Source: CAD feature listing. Evaluate the final solid. Frame: model axes, mm. A direction names the side the tool comes from. Give positions to 0.01 mm unless a question says otherwise; leave off trailing zeros. Write each loop counter-clockwise with the first axis right and the second up, starting at its lowest first coordinate (ties: lowest second). Pieces come first, ordered by that corner, then holes. Notation, with made-up numbers: M 72.25,65.5 L 76.25,65.5 A33 cw 76.25,98.5 Z; hole C 47.5,-20.75 d8. An arc over 180 degrees is marked long. Return JSON: item names as keys, results as strings.
```python
from build123d import *

# Parameters (mm, degrees)
SKETCH1_W           = 110
SKETCH1_H           = 30
BOSS_EXTRUDE1_DEPTH = 12
FILLET2_R           = 8
SKETCH4_R           = 6.5
CUT_EXTRUDE1_DEPTH  = 67.870108383
SKETCH3_W           = 23
SKETCH3_H           = 13
CUT_EXTRUDE2_DEPTH  = 10
SKETCH5_W           = 32
SKETCH5_H           = 18
CUT_EXTRUDE3_DEPTH  = 1.5
FILLET4_R           = 3
SKETCH8_R           = 6.5
CUT_EXTRUDE4_DEPTH  = 63.574437799
SKETCH10_W          = 23
SKETCH10_H          = 13
CUT_EXTRUDE5_DEPTH  = 10
SKETCH12_W          = 32
SKETCH12_H          = 18
CUT_EXTRUDE6_DEPTH  = 1.5
FILLET5_R           = 3
SKETCH14_R          = 1
CUT_EXTRUDE7_DEPTH  = 4
SKETCH6_R           = 1
CUT_EXTRUDE8_DEPTH  = 5


with BuildPart() as part:
    # Sketch1 → Boss-Extrude1 (new body)
    with BuildSketch(Plane(origin=(0, 0, 0), x_dir=(1, 0, 0), z_dir=(0, 1, 0))):
        with Locations((8.243243243, 3.108108108)):
            Rectangle(SKETCH1_W, SKETCH1_H)
    extrude(amount=BOSS_EXTRUDE1_DEPTH)

    # Fillet2
    fillet2_edges = [part.edges().sort_by_distance(p)[0] for p in [
        (-46.756756757, 6, -18.108108108),
        (63.243243243, 6, -18.108108108),
        (63.243243243, 6, 11.891891892),
        (-46.756756757, 6, 11.891891892),
    ]]
    fillet(fillet2_edges, radius=FILLET2_R)

    # Sketch4 → Cut-Extrude1 (cut, through all)
    with BuildSketch(Plane(origin=(0, 12, 0), x_dir=(1, 0, 0), z_dir=(0, 1, 0))):
        with Locations(Location((-27.929103529, 3.108108108, 0), (0, 0, 270))):
            Circle(SKETCH4_R)
    extrude(amount=-CUT_EXTRUDE1_DEPTH, mode=Mode.SUBTRACT)

    # Sketch3 → Cut-Extrude2 (cut)
    with BuildSketch(Plane(origin=(0, 12, 0), x_dir=(1, 0, 0), z_dir=(0, 1, 0))):
        with Locations((-23.179103529, 3.108108108)):
            Rectangle(SKETCH3_W, SKETCH3_H)
    extrude(amount=-CUT_EXTRUDE2_DEPTH, mode=Mode.SUBTRACT)

    # Sketch5 → Cut-Extrude3 (cut)
    with BuildSketch(Plane(origin=(0, 12, 0), x_dir=(1, 0, 0), z_dir=(0, 1, 0))):
        with Locations((-23.262280593, 3.273133416)):
            Rectangle(SKETCH5_W, SKETCH5_H)
    extrude(amount=-CUT_EXTRUDE3_DEPTH, mode=Mode.SUBTRACT)

    # Fillet4
    fillet4_edges = [part.edges().sort_by_distance(p)[0] for p in [
        (-39.262280593, 11.25, 5.726866584),
        (-39.262280593, 11.25, -12.273133416),
        (-7.262280593, 11.25, -12.273133416),
        (-7.262280593, 11.25, 5.726866584),
    ]]
    fillet(fillet4_edges, radius=FILLET4_R)

    # Sketch8 → Cut-Extrude4 (cut, through all)
    with BuildSketch(Plane(origin=(11.720616789, 0, 0.652410252), x_dir=(-1, 0, 0), z_dir=(0, -1, 0))):
        with Locations(Location((-27.929103529, 3.108108108, 0), (0, 0, 90))):
            Circle(SKETCH8_R)
    extrude(amount=-CUT_EXTRUDE4_DEPTH, mode=Mode.SUBTRACT)

    # Sketch10 → Cut-Extrude5 (cut)
    with BuildSketch(Plane(origin=(11.720616789, 0, 0.652410252), x_dir=(-1, 0, 0), z_dir=(0, -1, 0))):
        with Locations((-23.179103529, 3.108108108)):
            Rectangle(SKETCH10_W, SKETCH10_H)
    extrude(amount=-CUT_EXTRUDE5_DEPTH, mode=Mode.SUBTRACT)

    # Sketch12 → Cut-Extrude6 (cut)
    with BuildSketch(Plane(origin=(11.720616789, 0, 0.652410252), x_dir=(-1, 0, 0), z_dir=(0, -1, 0))):
        with Locations((-23.262280593, 3.273133416)):
            Rectangle(SKETCH12_W, SKETCH12_H)
    extrude(amount=-CUT_EXTRUDE6_DEPTH, mode=Mode.SUBTRACT)

    # Fillet5
    fillet5_edges = [part.edges().sort_by_distance(p)[0] for p in [
        (50.982897382, 0.75, 6.379276835),
        (50.982897382, 0.75, -11.620723165),
        (18.982897382, 0.75, -11.620723165),
        (18.982897382, 0.75, 6.379276835),
    ]]
    fillet(fillet5_edges, radius=FILLET5_R)

    # Sketch14 → Cut-Extrude7 (cut)
    with BuildSketch(Plane(origin=(11.720616789, 1.5, 0.652410252), x_dir=(-1, 0, 0), z_dir=(0, -1, 0))):
        with Locations(Location((-37.179103529, 3.108108108, 0), (0, 0, 90))):
            Circle(SKETCH14_R)
        with Locations(Location((-9.179103529, 3.108108108, 0), (0, 0, 270))):
            Circle(SKETCH14_R)
    extrude(amount=-CUT_EXTRUDE7_DEPTH, mode=Mode.SUBTRACT)

    # Sketch6 → Cut-Extrude8 (cut)
    with BuildSketch(Plane(origin=(0, 10.5, 0), x_dir=(1, 0, 0), z_dir=(0, 1, 0))):
        with Locations(Location((-37.179103529, 3.108108108, 0), (0, 0, 270))):
            Circle(SKETCH6_R)
        with Locations(Location((-9.179103529, 3.108108108, 0), (0, 0, 90))):
            Circle(SKETCH6_R)
    extrude(amount=-CUT_EXTRUDE8_DEPTH, mode=Mode.SUBTRACT)


solid = part.part
```
1) Cut plane C-C, the plane z = -6.5. Return the cut outline in (x, y).
Numbers:
{"outline": "M -46.76,0 L -33.47,0 L -33.47,2 L -34.68,2 L -34.68,10.5 L -39.26,10.5 L -39.26,12 L -46.76,12 Z; M -22.38,0 L 18.98,0 L 18.98,1.5 L 23.4,1.5 L 23.4,10 L 34.56,10 L 34.56,12 L -7.26,12 L -7.26,10.5 L -11.68,10.5 L -11.68,2 L -22.38,2 Z; M 44.74,10 L 46.4,10 L 46.4,1.5 L 50.98,1.5 L 50.98,0 L 63.24,0 L 63.24,12 L 44.74,12 Z"}
2) Set-up query: faces 5 (the face through (-10.02, 8.04, -3.65)), 6 (the face through (49, 5.5, -2)), 7 (the face through (33.304, 10.986, -1.047)). Return all of +Z, -Z, +X, -X, +Y, -Y with unobstructed straight access to the full face (end or side cutting, diameter ignored); none if empty.
Numbers:
{"face 5": "+Y", "face 6": "-Y", "face 7": "+Y, -Y"}
3) Cut plane D-D, the plane x = -30. Return the cut outline in (y, z), then the cut area to 3 significant figures.
Numbers:
{"outline": "M 0,-18.11 L 12,-18.11 L 12,-12.27 L 10.5,-12.27 L 10.5,-9.61 L 2,-9.61 L 2,-9.27 L 0,-9.27 Z; M 0,3.05 L 2,3.05 L 2,3.39 L 10.5,3.39 L 10.5,5.73 L 12,5.73 L 12,11.89 L 0,11.89 Z", "area": "198 mm²"}
4) Line query: line 1 (X direction, y = 3.5, z = 2); line 2 (X direction, y = 1.75, z = 0); line 3 (Z direction, x = -13, y = 11.75). Output: solid intervals per line, ascending. Write a range as [from, to].
Numbers:
{"line 1": "x = [-46.76, -34.68], [-11.68, 23.4], [46.4, 63.24]", "line 2": "x = [-46.76, -33.64], [-22.22, 23.4], [46.4, 63.24]", "line 3": "z = [-18.11, -12.27], [5.73, 11.89]"}
5) Contact query for flat-ended pins moving along their axis: pin 1 Ø17 at (x, z) = (39.65, -2.46) entering from -Y; pin 2 Ø1 at (x, z) = (-9.5, -3) entering from +Y; pin 3 Ø2 at (x, z) = (-33, 0) entering from +Y. Output: stop coordinate, or through.
Numbers:
{"pin 1": "stops at y = 1.5", "pin 2": "stops at y = 5.5", "pin 3": "stops at y = 2"}
6) Draft query along Z for faces 1 (the face through (60.84, 6.08, 9.61)), 2 (the face through (-8.118, 11.24, -11.371)), 3 (the face through (-38.36, 11.24, 4.87)), 4 (the face through (60.962, 6.084, -15.702)). Return one class per face: released by +Z, released by -Z, zero draft, split by the parting line, or undercut.
Numbers:
{"face 1": "released by +Z", "face 2": "undercut", "face 3": "undercut", "face 4": "released by -Z"}
7) Cut plane A-A, the plane x = 27. Return the cut outline in (y, z), then the cut area to 4 significant figures.
Numbers:
{"outline": "M 0,-18.11 L 12,-18.11 L 12,11.89 L 0,11.89 L 0,6.38 L 1.5,6.38 L 1.5,4.04 L 10,4.04 L 10,-8.96 L 1.5,-8.96 L 1.5,-11.62 L 0,-11.62 Z", "area": "222.5 mm²"}
8) Cut plane B-B, the plane y = 8.25. Return the cut outline in (x, z).
Numbers:
{"outline": "M -46.76,-10.11 A8 ccw -38.76,-18.11 L 55.24,-18.11 A8 ccw 63.24,-10.11 L 63.24,3.89 A8 ccw 55.24,11.89 L -38.76,11.89 A8 ccw -46.76,3.89 Z; hole C -37.18,-3.11 d2; hole M -34.68,-9.61 L -11.68,-9.61 L -11.68,3.39 L -34.68,3.39 Z; hole C -9.18,-3.11 d2; hole M 23.4,-8.96 L 46.4,-8.96 L 46.4,4.04 L 23.4,4.04 Z"}
